from build123d import *

# Parameters (mm, degrees)
ESQUISSE1_R             = 50
ESQUISSE1_R_2           = 40
BOSS_EXTRU_1_DEPTH      = 10
ESQUISSE2_R             = 48
ESQUISSE2_R_2           = 43
ENL_V_MAT_EXTRU_1_DEPTH = 0.5
ESQUISSE3_R             = 48
ESQUISSE3_R_2           = 43
ENL_V_MAT_EXTRU_2_DEPTH = 0.5
CONG_1_R                = 0.3


with BuildPart() as part:
    # Esquisse1 → Boss.-Extru.1 (new body)
    with BuildSketch(Plane.XY):
        Circle(ESQUISSE1_R)
        Circle(ESQUISSE1_R_2, mode=Mode.SUBTRACT)
    extrude(amount=BOSS_EXTRU_1_DEPTH)

    # Esquisse2 → Enlèv. mat.-Extru.1 (cut)
    with BuildSketch(Plane.XY.offset(10)):
        Circle(ESQUISSE2_R)
        Circle(ESQUISSE2_R_2, mode=Mode.SUBTRACT)
    extrude(amount=-ENL_V_MAT_EXTRU_1_DEPTH, mode=Mode.SUBTRACT)

    # Esquisse3 → Enlèv. mat.-Extru.2 (cut)
    with BuildSketch(Plane(origin=(0, 0, 0), x_dir=(-1, 0, 0), z_dir=(0, 0, -1))):
        Circle(ESQUISSE3_R)
        Circle(ESQUISSE3_R_2, mode=Mode.SUBTRACT)
    extrude(amount=-ENL_V_MAT_EXTRU_2_DEPTH, mode=Mode.SUBTRACT)

    # Congé1
    cong_1_edges = [part.edges().sort_by_distance(p)[0] for p in [
        (-50, 0, 0),
        (-50, 0, 10),
        (-40, 0, 0),
        (-40, 0, 10),
    ]]
    fillet(cong_1_edges, radius=CONG_1_R)


solid = part.part
The model under review builds one solid part; all positions refer to its coordinate system, in mm. A direction names the side the tool comes from. Give positions to 0.01 mm unless a question says otherwise; leave off trailing zeros. Loops run counter-clockwise (first coordinate to the right, second up) from the corner with the lowest first, then second, coordinate; pieces in that order, holes last. Notation, with made-up numbers: (14, 24) -> (59, 24) arc R18 ccw to (59, 30) -> close; hole circle Ø8 at (46.5, 59.25). An arc over 180 degrees is marked (long way). Answer as a JSON object with one key per item and string values. Group by question number.
Q1. Tool access review of faces 1 (the cylindrical face through (5.598, 42.634, 0.246)), 2 (the cylindrical face through (-47.954, 2.11, 9.754)), 3 (the cylindrical face through (-8.67, -39.05, 4.93)): name each direction out of +Z, -Z, +X, -X, +Y, -Y from which nothing blocks a thin tool from reaching the whole face with its end or side.
Q2. Insertion check: pin 1 (6 mm diameter, centred on x = -19.5, z = 6, fed in from +Y); pin 2 (4 mm diameter, centred on x = -32.5, z = 3.5, fed in from -Y); pin 3 (4 mm diameter, centred on x = 8.5, z = 7.5, fed in from -Y). Each pin has a flat end and moves straight along its axis. Give the tip position at first contact, or say it passes through.
Q3. Draft analysis for pull direction X (two halves, no side actions). For faces 4 (the flat face through (-39.3, 18, 9.5)), 5 (the flat face through (-41, 26, 0)), 6 (the cylindrical face through (47.69, 15.02, 4.93)), state which applies: pulls with the +X half, pulls with the -X half, needs draft (parallel to the pull), parting line crosses it, or undercut.
Q4. Wall thickness on line 1 along X through (y, z) = (1.5, 9.75); line 2 along Y through (x, z) = (0, 0.15); line 3 along Z through (x, y) = (38.5, 26): over which ranges is each line inside the solid? List them lowest first.
Q5. Take a section at C-C (z = 6.25). Write out the cut boundary in (x, y), plus the area to 3 significant figures.
Answer below:
{
 "1": {"face 1": "-Z", "face 2": "+Z", "face 3": "+Z, -Z"},
 "2": {"pin 1": "stops at y = 47.2", "pin 2": "stops at y = -39.62", "pin 3": "stops at y = -49.58"},
 "3": {"face 4": "undercut", "face 5": "needs draft", "face 6": "parting line crosses it"},
 "4": {"line 1": "x = -49.97 to -47.98, -42.97 to -39.98, 39.98 to 42.97, 47.98 to 49.97", "line 2": "y = -49.96 to -48, -43 to -40.04, 40.04 to 43, 48 to 49.96", "line 3": "z = 0.5 to 9.5"},
 "5": {"outline": "circle Ø100 at (0, 0); hole circle Ø80 at (0, 0)", "area": "2,830 mm2"}
}
